from build123d import *

# Parameters (mm, degrees)
BOSS_EXTRUDE1_DEPTH = 16
SKETCH4_R           = 6.5
CUT_EXTRUDE1_DEPTH  = 11
SKETCH5_R           = 3.45
CUT_EXTRUDE2_DEPTH  = 11
FILLET1_R           = 1


with BuildPart() as part:
    # Sketch3 → Boss-Extrude1 (new body)
    with BuildSketch(Plane.XY):
        Polygon((0, 0), (0, -32), (25, -32), (32.331439149, -22.5), (32.331439149, -9.5), (25, 0), align=None)
    extrude(amount=BOSS_EXTRUDE1_DEPTH)

    # Sketch4 → Cut-Extrude1 (cut)
    with BuildSketch(Plane.XY.offset(16)):
        with Locations((16.165719575, -16)):
            Circle(SKETCH4_R)
    extrude(amount=-CUT_EXTRUDE1_DEPTH, mode=Mode.SUBTRACT)

    # Sketch5 → Cut-Extrude2 (cut)
    with BuildSketch(Plane.XY.offset(5)):
        with Locations((16.165719575, -16)):
            Circle(SKETCH5_R)
    extrude(amount=-CUT_EXTRUDE2_DEPTH, mode=Mode.SUBTRACT)

    # Fillet1
    fillet1_edges = [part.edges().sort_by_distance(p)[0] for p in [
        (25, 0, 8),
        (32.331439149, -9.5, 8),
        (32.331439149, -22.5, 8),
        (25, -32, 8),
        (0, -32, 8),
        (0, 0, 8),
        (12.5, -32, 16),
        (28.665719575, -27.25, 16),
        (32.331439149, -16, 16),
        (9.665719575, -16, 5),
        (9.665719575, -16, 16),
        (28.665719575, -4.75, 16),
        (12.5, 0, 16),
        (28.665719575, -4.75, 0),
        (32.331439149, -16, 0),
        (28.665719575, -27.25, 0),
        (12.5, -32, 0),
        (0, -16, 0),
        (12.5, 0, 0),
        (0, -16, 16),
    ]]
    fillet(fillet1_edges, radius=FILLET1_R)


solid = part.part
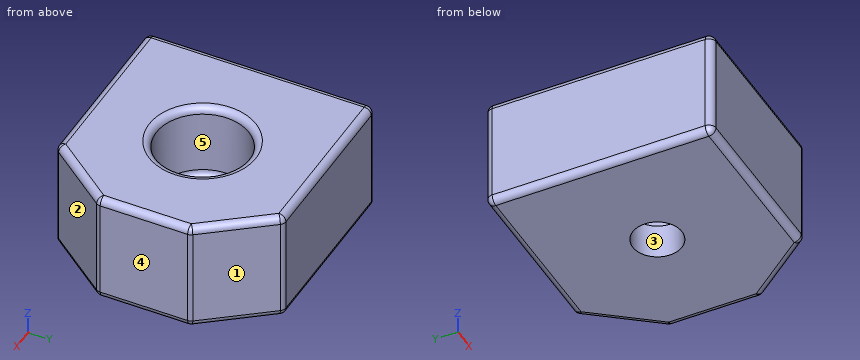
Source: CAD feature listing. Evaluate the final solid. Frame: model axes, mm. Face numbers are marked on the shaded views. A direction names the side the tool comes from. Round coordinates to 2 decimals unless told otherwise and drop trailing zeros. Loops run counter-clockwise (first coordinate to the right, second up) from the corner with the lowest first, then second, coordinate; pieces in that order, holes last. Notation, with made-up numbers: (15, -0.5) - (43, -0.5) arc R26 cw to (43, 24.5) - close; hole circle Ø10 at (26, 81). An arc over 180 degrees is marked (long way). Write item = value, one per line. Start each with the question number.
Item 1: Reachability of the marked faces 4 and 5 from +Z, -Z, +X, -X, +Y, -Y: full face, straight path, thin tool, end or side. Return the list, or none.
Item 2: Section query A-A on y = -16. Output: boundary loops of the cut face in (x, z).
Item 3: Section query C-C on z = 7.75. Output: boundary loops of the cut face in (x, y).
Item 4: Mould query, pull axis Y, two halves, no side actions, for the marked faces 1, 2 and 3. Classes: released by +Y, released by -Y, zero draft, split by the parting line, or undercut.
Item 5: Material intervals for line 1 (X direction, y = -18, z = 11.5); line 2 (Y direction, x = 15.5, z = 8.75); line 3 (X direction, y = -19, z = 6), sorted ascending.
Item 6: First-contact query: pin 1 Ø3.5 at (x, y) = (19, -18) entering from +Z; pin 2 Ø3 at (y, z) = (-26, 9.5) entering from +X. Flat tips, straight axial feed; report the tip coordinate or a pass-through.
Item 7: Section query B-B on z = 2. Output: boundary loops of the cut face in (x, y), plus the area to 3 significant figures.
Results list:
q1.face_4 = +Z, -Z, +X, +Y, -Y
q1.face_5 = +Z
q2.outline = (0, 1) arc R1 ccw to (1, 0) - (12.72, 0) - (12.72, 5) - (10.67, 5) arc R1 cw to (9.67, 6) - (9.67, 15) arc R1 ccw to (8.67, 16) - (1, 16) arc R1 ccw to (0, 15) - close; (19.62, 0) - (31.33, 0) arc R1 ccw to (32.33, 1) - (32.33, 15) arc R1 ccw to (31.33, 16) - (23.67, 16) arc R1 ccw to (22.67, 15) - (22.67, 6) arc R1 cw to (21.67, 5) - (19.62, 5) - close
q3.outline = (0, -31) arc R1 ccw to (1, -32) - (24.51, -32) arc R1 ccw to (25.3, -31.61) - (32.12, -22.77) arc R1 ccw to (32.33, -22.16) - (32.33, -9.84) arc R1 ccw to (32.12, -9.23) - (25.3, -0.39) arc R1 ccw to (24.51, 0) - (1, 0) arc R1 ccw to (0, -1) - close; hole circle Ø13 at (16.17, -16)
q4.face_1 = released by +Y
q4.face_2 = released by -Y
q4.face_3 = undercut
q5.line_1 = 0 to 9.98, 22.35 to 32.33
q5.line_2 = -32 to -22.47, -9.53 to 0
q5.line_3 = 0 to 10.4, 21.93 to 32.33
q6.pin_1 = 5
q6.pin_2 = 30.79
q7.outline = (0, -31) arc R1 ccw to (1, -32) - (24.51, -32) arc R1 ccw to (25.3, -31.61) - (32.12, -22.77) arc R1 ccw to (32.33, -22.16) - (32.33, -9.84) arc R1 ccw to (32.12, -9.23) - (25.3, -0.39) arc R1 ccw to (24.51, 0) - (1, 0) arc R1 ccw to (0, -1) - close; hole circle Ø6.9 at (16.17, -16)
q7.area = 927 mm²
